The drawing under review shows one solid part. Ordinate dimensions are in mm from its lowest x, y, z. Round coordinates to 2 decimals unless told otherwise and drop trailing zeros. Order: outer loops, then holes, each group sorted by start corner. A loop starts at its lowest first (then second) coordinate and runs counter-clockwise, first axis right, second up. Notation, with made-up numbers: (-2, -36) -> (41, -36) arc R24 cw to (41, -17) -> close; hole circle Ø7 at (-19, -8). An arc over 180 degrees is marked (long way). Use a Markdown table: item, result. Add a question column.
1) Consider section D-D (z = 59). State the section outline as (x, y) points, plus the area to 3 significant figures.
2) Clearance check with flat-ended pins moving along their axes: P1, Ø0.7, axis at x = 1.5, z = 27.5, coming from the -Y side; P2, Ø0.7, axis at x = 1.5, y = 115, coming from the -Z side; P3, Ø1.2, axis at x = 1, z = 62, coming from the +Y side. State where each tip first meets the part, or that it passes through.
3) Consider section B-B (z = 100). State the section outline as (x, y) points, plus the area to 3 significant figures.
4) Wall thickness on line 1 along Z through (x, y) = (0.85, 42); line 2 along Y through (x, z) = (1.95, 59); line 3 along Z through (x, y) = (2.25, 48.5): over which ranges is each line inside the solid? List them lowest first. Write a range as [from, to].
5) Consider section A-A (y = 42). State the section outline as (x, z) points.
6) Consider section C-C (x = 0.4). State the section outline as (y, z) points.
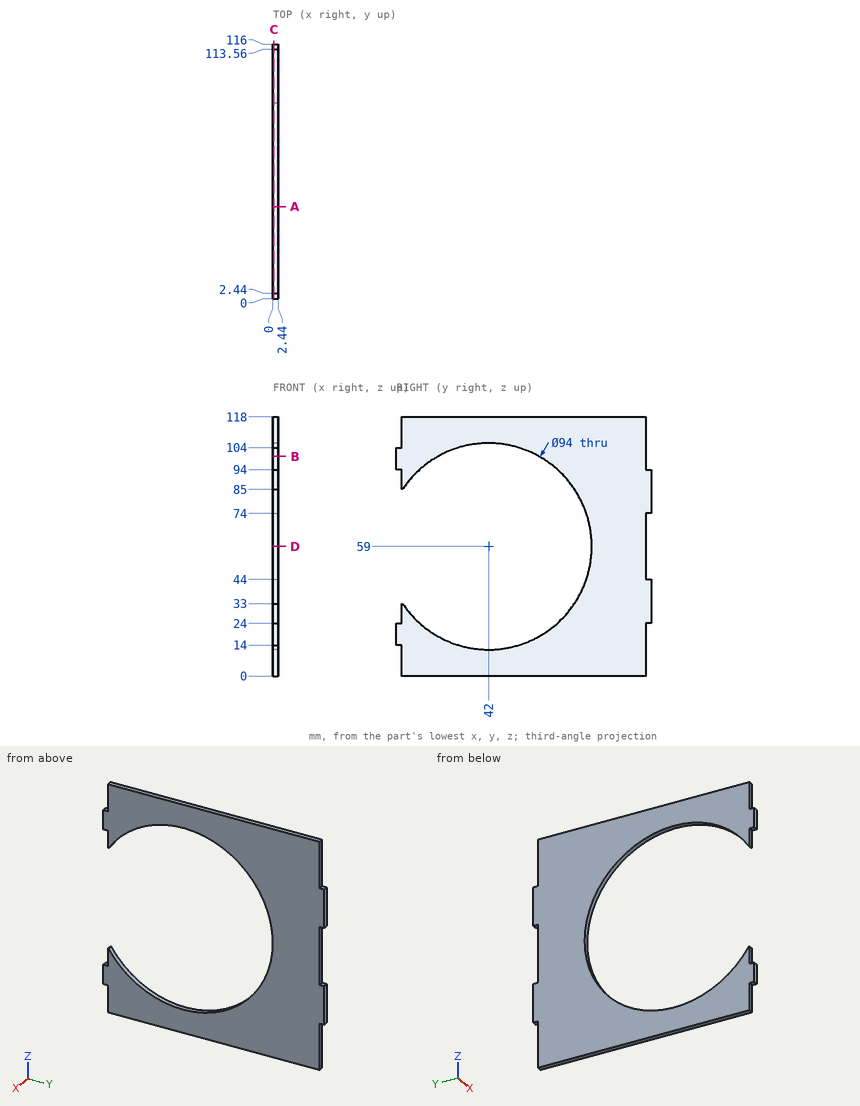
Results list:
| question | item | result |
|---|---|---|
| 1 | outline | (0, 89) -> (2.44, 89) -> (2.44, 113.56) -> (0, 113.56) -> close |
| 1 | area | 59.9 mm2 |
| 2 | P1 | y = 2.44 |
| 2 | P2 | z = 24 |
| 2 | P3 | y = 113.56 |
| 3 | outline | (0, 0) -> (2.44, 0) -> (2.44, 19.02) -> (0, 19.02) -> close; (0, 64.98) -> (2.44, 64.98) -> (2.44, 113.56) -> (0, 113.56) -> close |
| 3 | area | 165 mm2 |
| 4 | line 1 | [0, 12], [106, 118] |
| 4 | line 2 | [89, 113.56] |
| 4 | line 3 | [0, 12.45], [105.55, 118] |
| 5 | outline | (0, 0) -> (2.44, 0) -> (2.44, 12) -> (0, 12) -> close; (0, 106) -> (2.44, 106) -> (2.44, 118) -> (0, 118) -> close |
| 6 | outline | (0, 14) -> (2.44, 14) -> (2.44, 0) -> (113.56, 0) -> (113.56, 24) -> (116, 24) -> (116, 44) -> (113.56, 44) -> (113.56, 74) -> (116, 74) -> (116, 94) -> (113.56, 94) -> (113.56, 118) -> (2.44, 118) -> (2.44, 104) -> (0, 104) -> (0, 94) -> (2.44, 94) -> (2.44, 85) -> (2.85, 85) arc R47 cw (long way) to (2.85, 33) -> (2.44, 33) -> (2.44, 24) -> (0, 24) -> close |
